The model under review builds one solid part; all positions refer to its coordinate system, in mm. A direction names the side the tool comes from. Round coordinates to 2 decimals unless told otherwise and drop trailing zeros. Write each loop counter-clockwise with the first axis right and the second up, starting at its lowest first coordinate (ties: lowest second). Pieces come first, ordered by that corner, then holes. Notation, with made-up numbers: (84, 77) -> (111, 77) arc R20 ccw to (111, 98) -> close; hole circle Ø7 at (-40, -4). An arc over 180 degrees is marked (long way). Answer as a JSON object with one key per item and string values. Group by question number.
1) Insertion check: pin 1 Ø1 at (y, z) = (-1, 3) entering from +X; pin 2 Ø2 at (y, z) = (3.5, 3.5) entering from -X. Each pin has a flat end and moves straight along its axis. Give the tip position at first contact, or say it passes through.
2) We need section C-C, the plane y = -0.75. Write out the cut boundary in (x, z), then the cut area to 3 significant figures.
3) We need section A-A, the plane z = 2.5. Write out the cut boundary in (x, y).
4) To check wall thickness, follow probe 1 along X at (y, z) = (-4.35, 2.5); probe 2 along Z at (x, y) = (9.5, -4.4); probe 3 along X at (y, z) = (0, 2.6). State the ranges of each line that lie inside material, in increasing order. Write a range as [from, to].
5) Machinability: for faces 5 (the flat face through (-12, -4, 2)), 6 (the flat face through (-3.571, -4, 2)), 7 (the flat face through (11, -2.5, 4)), 8 (the cylindrical face through (0, 5, 2)), 9 (the flat face through (-11, -2.5, 4)), which of the approach directions +Z, -Z, +X, -X, +Y, -Y give a long, thin tool a straight path to every point of the face, cutting with its end or side? Answer none if there is none.
6) Mouldability with a two-part tool opening along Z and no side actions: class faces 1 (the flat face through (7.8, -5.5, 2.5)), 2 (the cylindrical face through (-7, 0.6, 2.5)), 3 (the flat face through (3, 5, 0)), 4 (the cylindrical face through (8.39, -3.98, 1.49)) as pulls with the +Z half, pulls with the -Z half, needs draft (parallel to the pull), parting line crosses it, or undercut.
7) We need section B-B, the plane x = 9.5. Write out the cut boundary in (y, z), then the cut area to 3 significant figures.
8) We need section D-D, the plane z = 1.25. Write out the cut boundary in (x, y), then the cut area to 3 significant figures.
from build123d import *

# Parameters (mm, degrees)
RESSALTO_EXTRUS_O1_DEPTH   = 5
ESBO_O2_R                  = 1.5
CORTE_EXTRUS_O1_DEPTH      = 12.5
CORTE_EXTRUS_O1_DEPTH_BACK = 4
ESBO_O3_R                  = 2.5
CORTE_EXTRUS_O2_DEPTH      = 12.5000001


with BuildPart() as part:
    # Esboço1 → Ressalto-extrusão1 (new body)
    with BuildSketch(Plane.XY):
        with BuildLine():
            Line((-9, -2.5), (-9, 0))
            ThreePointArc((-9, 0), (0, 9), (9, 0))
            Line((9, 0), (9, -2.5))
            Line((9, -2.5), (12, -2.5))
            Line((12, -2.5), (12, -5.5))
            Line((12, -5.5), (3.570714214, -5.5))
            Line((3.570714214, -5.5), (3.570714214, -3.5))
            ThreePointArc((3.570714214, -3.5), (0, 5), (-3.570714214, -3.5))
            Line((-3.570714214, -3.5), (-3.570714214, -5.5))
            Line((-3.570714214, -5.5), (-12, -5.5))
            Line((-12, -5.5), (-12, -2.5))
            Line((-12, -2.5), (-9, -2.5))
        make_face()
    extrude(amount=RESSALTO_EXTRUS_O1_DEPTH)

    # Esboço2 → Corte-extrusão1 (cut, two sides)
    with BuildSketch(Plane(origin=(0, -2.5, 0), x_dir=(1, 0, 0), z_dir=(0, 1, 0))) as corte_extrus_o1_sk:
        with Locations((-9.5, -2.5)):
            Circle(ESBO_O2_R)
        with Locations((9.5, -2.5)):
            Circle(ESBO_O2_R)
    extrude(amount=CORTE_EXTRUS_O1_DEPTH, mode=Mode.SUBTRACT)
    extrude(corte_extrus_o1_sk.sketch, amount=-CORTE_EXTRUS_O1_DEPTH_BACK, mode=Mode.SUBTRACT)

    # Esboço3 → Corte-extrusão2 (cut, through all)
    with BuildSketch(Plane(origin=(0, -2.5, 0), x_dir=(1, 0, 0), z_dir=(0, 1, 0))):
        with Locations((-9.5, -2.5)):
            Circle(ESBO_O3_R)
        with Locations((9.5, -2.5)):
            Circle(ESBO_O3_R)
    extrude(amount=CORTE_EXTRUS_O2_DEPTH, mode=Mode.SUBTRACT)


solid = part.part
Here are the results:
{
 "1": {"pin 1": "stops at x = 7.21", "pin 2": "stops at x = -8"},
 "2": {"outline": "(-9, 0) -> (-4.94, 0) -> (-4.94, 5) -> (-9, 5) -> (-9, 4.95) arc R2.5 cw to (-9, 0.05) -> close; (4.94, 0) -> (9, 0) -> (9, 0.05) arc R2.5 cw to (9, 4.95) -> (9, 5) -> (4.94, 5) -> close", "area": "25.9 mm^2"},
 "3": {"outline": "(-12, -5.5) -> (-11, -5.5) -> (-11, -2.5) -> (-12, -2.5) -> close; (-8, -5.5) -> (-3.57, -5.5) -> (-3.57, -3.5) arc R5 cw (long way) to (3.57, -3.5) -> (3.57, -5.5) -> (8, -5.5) -> (8, -2.5) -> (7, -2.5) -> (7, 5.66) arc R9 ccw to (-7, 5.66) -> (-7, -2.5) -> (-8, -2.5) -> close; (11, -5.5) -> (12, -5.5) -> (12, -2.5) -> (11, -2.5) -> close"},
 "4": {"probe 1": "x = [-12, -11], [-8, -3.57], [3.57, 8], [11, 12]", "probe 2": "z = [0, 1], [4, 5]", "probe 3": "x = [-7, -5], [5, 7]"},
 "5": {"face 5": "+Z, -Z, -X, +Y, -Y", "face 6": "+Z, -Z, -Y", "face 7": "+X, +Y", "face 8": "+Z, -Z", "face 9": "-X, +Y"},
 "6": {"face 1": "needs draft", "face 2": "undercut", "face 3": "pulls with the -Z half", "face 4": "undercut"},
 "7": {"outline": "(-5.5, 0) -> (-2.5, 0) -> (-2.5, 1) -> (-5.5, 1) -> close; (-5.5, 4) -> (-2.5, 4) -> (-2.5, 5) -> (-5.5, 5) -> close", "area": "6.00 mm^2"},
 "8": {"outline": "(-12, -5.5) -> (-10.33, -5.5) -> (-10.33, -2.5) -> (-12, -2.5) -> close; (-8.67, -5.5) -> (-3.57, -5.5) -> (-3.57, -3.5) arc R5 cw (long way) to (3.57, -3.5) -> (3.57, -5.5) -> (8.67, -5.5) -> (8.67, -2.5) -> (7.33, -2.5) -> (7.33, 5.22) arc R9 ccw to (-7.33, 5.22) -> (-7.33, -2.5) -> (-8.67, -2.5) -> close; (10.33, -5.5) -> (12, -5.5) -> (12, -2.5) -> (10.33, -2.5) -> close", "area": "129 mm^2"}
}
